Work out the finished part from the listing and answer in its coordinate system (mm). A direction names the side the tool comes from. Round coordinates to 2 decimals unless told otherwise and drop trailing zeros. Order: outer loops, then holes, each group sorted by start corner. A loop starts at its lowest first (then second) coordinate and runs counter-clockwise, first axis right, second up. Notation, with made-up numbers: M 27,11 L 71,11 A23 ccw 71,32 Z; hole C 28,28 d6. An arc over 180 degrees is marked long. Return JSON: item names as keys, results as strings.
Autodesk Inventor part; units mm, degrees
ref_plane "YZ Plane" through (0, 0, 0) normal (1, 0, 0) x (0, 1, 0)
ref_plane "XZ Plane" through (0, 0, 0) normal (0, 1, 0) x (-1, 0, 0)
ref_plane "XY Plane" through (0, 0, 0) normal (0, 0, 1) x (1, 0, 0)
sketch "Sketch1" plane through (0, 0, 0) normal (0, 0, 1) x (1, 0, 0)
  line L0 (40, -40) -> (-40, -40)
  line L1 (-40, -40) -> (-40, 40)
  line L2 (-40, 40) -> (40, 40)
  line L3 (40, 40) -> (40, -40)
  line L4 (40, -40) -> (-40, 40) construction
  line L5 (-40, -40) -> (40, 40) construction
  circle A0 centre (0, 0) radius 57.5
  dimension "d0" = 80
  dimension "d72" = 115
extrude "Extrusion1" add sketch "Sketch1" along normal blind 10 contours L0 L1 L2 L3 | A0
sketch "Sketch2" plane through (0, 0, 0) normal (0, 0, -1) x (-1, 0, 0)
  arc A0 (40, 37) -> (37, 40) centre (37, 37) ccw
  line L0 (30.15, -30.15) -> (-30.15, -30.15)
  line L1 (-30.15, -30.15) -> (-30.15, 30.15)
  line L2 (-30.15, 30.15) -> (30.15, 30.15)
  line L3 (30.15, 30.15) -> (30.15, -30.15)
  line L4 (30.15, -30.15) -> (-30.15, 30.15) construction
  line L5 (-30.15, -30.15) -> (30.15, 30.15) construction
  circle A1 centre (-30.15, 30.15) radius 4.75
  circle A2 centre (30.15, 30.15) radius 4.75
  circle A3 centre (30.15, -30.15) radius 4.75
  circle A4 centre (-30.15, -30.15) radius 4.75
  point P0 (0, 0)
  point P1 (39.1213, 39.1213)
  dimension "d32" = 60.3
  dimension "d33" = 9.5
hole "Hole3" at (30.15, -30.15, 0) at (30.15, 30.15, 0) at (-30.15, 30.15, 0) at (-30.15, -30.15, 0) direction (0, 0, 1) diameter 6.6 end through all
sketch "Sketch3" plane through (0, 0, 0) normal (0, 0, -1) x (-1, 0, 0)
  circle A0 centre (0, 0) radius 40
  circle A1 centre (0, 40) radius 2.5
  circle A2 centre (40, 0) radius 2.5
  circle A3 centre (0, -40) radius 2.5
  circle A4 centre (-40, 0) radius 2.5
  circle A5 centre (-0.0779, 0.0489) radius 2.5
  dimension "d12" = 5
  dimension "d60" = 80
  dimension "d74" = 5
hole "Hole1" at (40, 0, 0) at (0, 40, 0) at (0, -40, 0) at (-40, 0, 0) at (0.0779, 0.0489, 0) direction (0, 0, 1) diameter 7 end through all
sketch "Sketch8" plane through (0, 0, 0) normal (0, 0, -1) x (-1, 0, 0)
  circle A0 centre (0, 0) radius 40
  circle A1 centre (0, 40) radius 12.0233
  circle A2 centre (40, 0) radius 12.001
  circle A3 centre (-40, 0) radius 12.185
  circle A4 centre (0, -40) radius 12.001
  circle A5 centre (-0.3746, -0.3656) radius 12.0233
  dimension "d61" = 80
hole "Hole4" at (-40, 0, 0) at (0, 40, 0) at (40, 0, 0) at (0, -40, 0) at (0.3746, -0.3656, 0) direction (0, 0, 1) diameter 20 depth 7
sketch "Sketch10" plane through (0, 0, 10) normal (0, 0, 1) x (1, 0, 0)
  circle A0 centre (30.15, 30.15) radius 3.3
  circle A1 centre (30.15, 30.15) radius 6
  circle A2 centre (-30.15, 30.15) radius 3.3
  circle A3 centre (-30.15, 30.15) radius 6
  circle A4 centre (-30.15, -30.2444) radius 6
  circle A5 centre (30.15, -30.2444) radius 6
  point P0 (0, 0)
  dimension "d63" = 12
hole "Hole5" at (-30.15, -30.2444, 10) at (30.15, -30.2444, 10) at (30.15, 30.15, 10) at (-30.15, 30.15, 10) direction (0, 0, -1) diameter 12 depth 7
properties part number "adaptor_spine_base"
Item 1: Find section C-C (z = 8.5). State how many separate pieces and enclosed holes the cut face has, plus the area to 3 significant figures.
Output:
{"separate pieces": "1", "enclosed holes": "9", "area": "9,740 mm^2"}
Item 2: Find section D-D (y = 0). Determine the outline of the cut face in (x, z), plus the area to 3 significant figures.
Output:
{"outline": "M -57.5,0 L -50,0 L -50,7 L -43.5,7 L -43.5,10 L -57.5,10 Z; M -36.5,7 L -30,7 L -30,0 L -9.62,0 L -9.62,7 L -3.42,7 L -3.42,10 L -36.5,10 Z; M 3.58,7 L 10.37,7 L 10.37,0 L 30,0 L 30,7 L 36.5,7 L 36.5,10 L 3.58,10 Z; M 43.5,7 L 50,7 L 50,0 L 57.5,0 L 57.5,10 L 43.5,10 Z", "area": "667 mm^2"}
Item 3: Consider line 1 along Y through (x, z) = (0, 4.5); line 2 along Y through (x, z) = (28.5, 4.5); line 3 along Z through (x, y) = (5, -5). Determine where each line is inside the solid, lowest interval first. Write a range as [from, to].
Output:
{"line 1": "y = [-57.5, -50], [-30, -10.36], [9.63, 30], [50, 57.5]", "line 2": "y = [-49.94, -36.01], [-24.48, 24.38], [35.92, 49.94]", "line 3": "z = [7, 10]"}
Item 4: Each of these flat-tipped pins is pushed along its axis until it touches: pin 1 (4 mm diameter, centred on x = -19.5, y = -22.5, fed in from -Z); pin 2 (8.5 mm diameter, centred on x = 30.15, y = 30.15, fed in from +Z); pin 3 (6 mm diameter, centred on y = -34.5, z = 6, fed in from -X); pin 4 (3 mm diameter, centred on x = -28.5, z = 6.5, fed in from +Y). Where does it stop, or does it pass through?
Output:
{"pin 1": "stops at z = 0", "pin 2": "stops at z = 3", "pin 3": "stops at x = -48.1", "pin 4": "stops at y = 50.77"}
Item 5: Find section A-A (x = -40). Determine the outline of the cut face in (y, z).
Output:
{"outline": "M -41.31,0 L -10,0 L -10,7 L -3.5,7 L -3.5,10 L -41.31,10 Z; M 3.5,7 L 10,7 L 10,0 L 41.31,0 L 41.31,10 L 3.5,10 Z"}
Item 6: The mould has two halves that part along Y. Classify faces 4 (the flat face through (12, 1, 10)), 5 (the flat face through (4, 40, 7)): pulls with the +Y half, pulls with the -Y half, needs draft (parallel to the pull), parting line crosses it, or undercut.
Output:
{"face 4": "needs draft", "face 5": "undercut"}
Item 7: Which of the six approach directions +Z, -Z, +X, -X, +Y, -Y give full straight-line access (tool end or side, diameter ignored) to faces 1 (the cylindrical face through (-30.24, -2.17, 3.55)), 2 (the cylindrical face through (-36.1, -29.46, 6.45)), 3 (the cylindrical face through (-0.154, 36.503, 8.521))?
Output:
{"face 1": "-Z", "face 2": "+Z", "face 3": "+Z, -Z"}
